Here's how the part is built. I have some questions about the finished solid (model axes, mm). A direction names the side the tool comes from. Coordinates: 2 decimals unless noted, no trailing zeros. Write each loop counter-clockwise with the first axis right and the second up, starting at its lowest first coordinate (ties: lowest second). Pieces come first, ordered by that corner, then holes. Notation, with made-up numbers: (23, 55) - (70, 55) arc R15 cw to (70, 70) - close; hole circle Ø1 at (-6, 13). An arc over 180 degrees is marked (long way). Answer in a Markdown table with one row per item. Add a question column.
Item 1: I'm going to push flat-ended pins straight in: pin 1 (6 mm diameter, centred on x = 35.2, y = -14.58, fed in from +Z) (3 decimals); pin 2 (3 mm diameter, centred on x = -8.5, z = 4, fed in from +Y); pin 3 (1 mm diameter, centred on x = 31, z = -9, fed in from +Y). Where does each tip first touch, or does it pass through?
Item 2: If I drill on probe 1 along Y at (x, z) = (-32, 54.5); probe 2 along Y at (x, z) = (-10, 1); probe 3 along Y at (x, z) = (-23, 53), over which ranges is the centre line in solid material (lowest first)? Write a range as from..to.
Item 3: Which directions (+Z, -Z, +X, -X, +Y, -Y) give clear straight access to the entire face, cutting with the end or side of a thin tool? Please do faces 1 (the face through (-8, 52, 57.15)), 2 (the face through (15, -35, 53.975)), 3 (the face through (-15.242, 30.163, -60.414)).
Item 4: We'd pull the mould along X, two halves only. Please class faces 4 (the face through (15, -35, -53.975)), 5 (the face through (-39.78, 36.48, -60.28)): +X half, -X half, draft (parallel to the pull), parting line (faces both ways), or undercut.
Item 5: Imagine slicing it at A-A (z = -36.5). Please give me the cut outline in (x, y) (3 decimals), plus the area to 3 significant figures.
Autodesk Inventor part; units mm, degrees
ref_plane "YZ Plane" through (0, 0, 0) normal (1, 0, 0) x (0, 1, 0)
ref_plane "XZ Plane" through (0, 0, 0) normal (0, 1, 0) x (-1, 0, 0)
ref_plane "XY Plane" through (0, 0, 0) normal (0, 0, 1) x (1, 0, 0)
sketch "Sketch1" plane through (0, 0, 0) normal (0, 0, 1) x (1, 0, 0)
  circle A0 centre (0, 0) radius 53.975
  dimension "d0" = 107.95
extrude "Extrusion1" add sketch "Sketch1" along normal mid plane 114.3
chamfer "Chamfer1" distance 1.5875 angle 45 1 edges at (-53.975, 0, 57.15)
chamfer "Chamfer2" distance 1.5875 angle 45 1 edges at (-53.975, 0, -57.15)
sketch "Sketch3" plane through (0, 0, 57.15) normal (0, 0, 1) x (1, 0, 0)
  circle A0 centre (0, 0) radius 53.975
extrude "Front End" add sketch "Sketch3" along normal blind 9.525
sketch "Sketch5" plane through (0, 0, 66.675) normal (0, 0, 1) x (1, 0, 0)
  circle A0 centre (0, 0) radius 53.975
  line L0 (0, 0) -> (31.4309, 31.4309) construction
  line L1 (-75.565, 0) -> (75.565, 0)
  line L2 (0, -75.565) -> (0, 75.565)
  point P0 (-31.4309, 31.4309)
  point P1 (-31.4309, -31.4309)
  point P2 (31.4309, -31.4309)
  dimension "d25" = 360
  dimension "d46" = 45
  dimension "d47" = 44.45
hole "Mount Holes" at (31.4309, 31.4309, 66.675) at (-31.4309, 31.4309, 66.675) at (-31.4309, -31.4309, 66.675) at (31.4309, -31.4309, 66.675) direction (0, 0, -1) diameter 3.683 depth 12.7 tip angle 118
sketch "Sketch6" plane through (0, 0, 66.675) normal (0, 0, 1) x (1, 0, 0)
  circle A0 centre (0, 0) radius 53.975
  circle A1 centre (0, 0) radius 6.35
  dimension "d34" = 12.7
extrude "Shaft Hole" cut sketch "Sketch6" against normal blind 12.7 contours A1
sketch "Sketch7" plane through (0, 0, 66.675) normal (0, 0, 1) x (1, 0, 0)
  circle A0 centre (0, 0) radius 6.35
  circle A1 centre (0, 0) radius 53.975
  circle A2 centre (35.1998, 14.5802) radius 5.08
  line L0 (0, 0) -> (35.1998, 14.5802) construction
  line L1 (0, -75.565) -> (0, 75.565)
  line L2 (-75.565, 0) -> (75.565, 0)
  circle A3 centre (14.5802, 35.1998) radius 5.08
  circle A4 centre (-14.5802, 35.1998) radius 5.08
  circle A5 centre (-35.1998, 14.5802) radius 5.08
  circle A6 centre (-35.1998, -14.5802) radius 5.08
  circle A7 centre (-14.5802, -35.1998) radius 5.08
  circle A8 centre (14.5802, -35.1998) radius 5.08
  circle A9 centre (35.1998, -14.5802) radius 5.08
  dimension "d37" = 10.16
  dimension "d38" = 22.5
  dimension "d39" = 38.1
  dimension "d42" = 360
extrude "Ventilation Holes" cut sketch "Sketch7" against normal blind 12.7 contours A2 | A3 | A4 | A5 | A6 | A7 | A8 | A9
mirror "Mirror3" about plane through (0, 0, 0) normal (0, 0, 1) of "Front End", "Mount Holes", "Ventilation Holes"
fillet "Fillet1" radius 3.175 2 edges at (-53.975, 0, 66.675) (-53.975, 0, -66.675)
properties part number "my1020_motor"
Here are the results:
| question | item | result |
|---|---|---|
| 1 | pin 1 | stops at z = 53.975 |
| 1 | pin 2 | stops at y = 53.52 |
| 1 | pin 3 | stops at y = 44.53 |
| 2 | probe 1 | y = -43.47..-33.18, -29.68..-18.53, -10.63..10.63, 18.53..29.68, 33.18..43.47 |
| 2 | probe 2 | y = -53.04..53.04 |
| 2 | probe 3 | y = -48.83..48.83 |
| 3 | face 1 | none |
| 3 | face 2 | +Z |
| 3 | face 3 | -Z |
| 4 | face 4 | undercut |
| 4 | face 5 | parting line |
| 5 | outline | circle Ø107.95 at (0, 0) |
| 5 | area | 9,150 mm2 |
